```python
from build123d import *

# Parameters (mm, degrees)
SKETCH1_W           = 6.45
SKETCH1_H           = 14.9
SKETCH1_R           = 2.69
BOSS_EXTRUDE1_DEPTH = 2
SKETCH1_4_R         = 1.2
BOSS_EXTRUDE2_DEPTH = 1.08
SKETCH2_R           = 2.69
BOSS_EXTRUDE3_DEPTH = 3.45
BOSS_EXTRUDE4_DEPTH = 3.45
BOSS_EXTRUDE5_DEPTH = 2.45
SKETCH2_5_R         = 3.5
SKETCH2_5_R_2       = 2.69
BOSS_EXTRUDE6_DEPTH = 3.45
SKETCH2_6_R         = 3.5
SKETCH2_6_R_2       = 2.69
BOSS_EXTRUDE7_DEPTH = 5.5


with BuildPart() as part:
    # Sketch1 → Boss-Extrude1 (new body)
    with BuildSketch(Plane(origin=(0, 0, 0), x_dir=(1, 0, 0), z_dir=(0, 1, 0))):
        with BuildLine():
            ThreePointArc((-7.492590556, 11.885435909), (-7.808434164, 9.098816182), (-10.610710111, 9.209523926))
            Line((-10.610710111, 9.209523926), (-11.865304556, 10.471159095))
            ThreePointArc((-11.865304556, 10.471159095), (-15.824865609, 0.065218614), (-11.951209075, -10.373004706))
            Line((-11.951209075, -10.373004706), (-10.610710111, -9.209523926))
            ThreePointArc((-10.610710111, -9.209523926), (-7.808434164, -9.098816182), (-7.492590556, -11.885435909))
            Line((-7.492590556, -11.885435909), (-8.439163385, -13.386976745))
            ThreePointArc((-8.439163385, -13.386976745), (0, -15.825), (8.439163385, -13.386976745))
            Line((8.439163385, -13.386976745), (7.492590556, -11.885435909))
            ThreePointArc((7.492590556, -11.885435909), (7.808434164, -9.098816182), (10.610710111, -9.209523926))
            Line((10.610710111, -9.209523926), (11.865304556, -10.471159095))
            ThreePointArc((11.865304556, -10.471159095), (14.802011174, -5.597418173), (15.825, 0))
            ThreePointArc((15.825, 0), (14.802011174, 5.597418173), (11.865304556, 10.471159095))
            Line((11.865304556, 10.471159095), (10.610710111, 9.209523926))
            ThreePointArc((10.610710111, 9.209523926), (7.808434164, 9.098816182), (7.492590556, 11.885435909))
            Line((7.492590556, 11.885435909), (8.549217648, 13.316962965))
            ThreePointArc((8.549217648, 13.316962965), (0, 15.825), (-8.549217648, 13.316962965))
            Line((-8.549217648, 13.316962965), (-7.492590556, 11.885435909))
        make_face()
        with Locations((-8.77, 0)):
            Rectangle(SKETCH1_W, SKETCH1_H, mode=Mode.SUBTRACT)
        with Locations(Location((0, 0, 0), (0, 0, 270))):
            Circle(SKETCH1_R, mode=Mode.SUBTRACT)
        with Locations((8.77, 0)):
            Rectangle(SKETCH1_W, SKETCH1_H, mode=Mode.SUBTRACT)
    extrude(amount=BOSS_EXTRUDE1_DEPTH)

    # Sketch1_4 → Boss-Extrude2 (add)
    with BuildSketch(Plane(origin=(0, 0, 0), x_dir=(1, 0, 0), z_dir=(0, 1, 0))):
        with BuildLine():
            Line((-10.610710111, -9.209523926), (-11.951209075, -10.373004706))
            ThreePointArc((-11.951209075, -10.373004706), (-10.305960854, -12.009071399), (-8.439163385, -13.386976745))
            Line((-8.439163385, -13.386976745), (-7.492590556, -11.885435909))
            ThreePointArc((-7.492590556, -11.885435909), (-7.808434164, -9.098816182), (-10.610710111, -9.209523926))
        make_face()
        with Locations(Location((-9.15, -10.662082348, 0), (0, 0, 270))):
            Circle(SKETCH1_4_R, mode=Mode.SUBTRACT)
        with BuildLine():
            Line((-11.865304556, 10.471159095), (-10.610710111, 9.209523926))
            ThreePointArc((-10.610710111, 9.209523926), (-7.808434164, 9.098816182), (-7.492590556, 11.885435909))
            Line((-7.492590556, 11.885435909), (-8.549217648, 13.316962965))
            ThreePointArc((-8.549217648, 13.316962965), (-10.305960854, 12.009071399), (-11.865304556, 10.471159095))
        make_face()
        with Locations(Location((-9.15, 10.662082348, 0), (0, 0, 270))):
            Circle(SKETCH1_4_R, mode=Mode.SUBTRACT)
        with BuildLine():
            ThreePointArc((11.865304556, 10.471159095), (10.305960854, 12.009071399), (8.549217648, 13.316962965))
            Line((8.549217648, 13.316962965), (7.492590556, 11.885435909))
            ThreePointArc((7.492590556, 11.885435909), (7.808434164, 9.098816182), (10.610710111, 9.209523926))
            Line((10.610710111, 9.209523926), (11.865304556, 10.471159095))
        make_face()
        with Locations(Location((9.15, 10.662082348, 0), (0, 0, 270))):
            Circle(SKETCH1_4_R, mode=Mode.SUBTRACT)
        with BuildLine():
            Line((7.492590556, -11.885435909), (8.439163385, -13.386976745))
            ThreePointArc((8.439163385, -13.386976745), (10.256381074, -12.051442746), (11.865304556, -10.471159095))
            Line((11.865304556, -10.471159095), (10.610710111, -9.209523926))
            ThreePointArc((10.610710111, -9.209523926), (7.808434164, -9.098816182), (7.492590556, -11.885435909))
        make_face()
        with Locations(Location((9.15, -10.662082348, 0), (0, 0, 270))):
            Circle(SKETCH1_4_R, mode=Mode.SUBTRACT)
    extrude(amount=BOSS_EXTRUDE2_DEPTH)

    # Sketch2_3 → Boss-Extrude4 (add)
    with BuildSketch(Plane(origin=(0, 0, 0), x_dir=(1, 0, 0), z_dir=(0, 1, 0))):
        with BuildLine():
            Line((-8.549217648, 13.316962965), (-7.692058181, 12.155676285))
            ThreePointArc((-7.692058181, 12.155676285), (0, 14.385), (7.692058181, 12.155676285))
            Line((7.692058181, 12.155676285), (8.549217648, 13.316962965))
            ThreePointArc((8.549217648, 13.316962965), (0, 15.825), (-8.549217648, 13.316962965))
        make_face()
        with BuildLine():
            ThreePointArc((7.671239513, -12.168825307), (0, -14.385), (-7.671239513, -12.168825307))
            Line((-7.671239513, -12.168825307), (-8.439163385, -13.386976745))
            ThreePointArc((-8.439163385, -13.386976745), (0, -15.825), (8.439163385, -13.386976745))
            Line((8.439163385, -13.386976745), (7.671239513, -12.168825307))
        make_face()
    extrude(amount=-BOSS_EXTRUDE4_DEPTH)

    # Sketch2_4 → Boss-Extrude5 (add)
    with BuildSketch(Plane(origin=(0, 0, 0), x_dir=(1, 0, 0), z_dir=(0, 1, 0))):
        with BuildLine():
            Line((-11.995, -2.98), (-11.995, -1.63))
            Line((-11.995, -1.63), (-14.292351976, -1.63))
            ThreePointArc((-14.292351976, -1.63), (-14.198702945, -2.307609084), (-14.072946564, -2.98))
            Line((-14.072946564, -2.98), (-11.995, -2.98))
        make_face()
        with BuildLine():
            Line((-11.995, 1.63), (-11.995, 2.98))
            Line((-11.995, 2.98), (-14.072946564, 2.98))
            ThreePointArc((-14.072946564, 2.98), (-14.198702945, 2.307609084), (-14.292351976, 1.63))
            Line((-14.292351976, 1.63), (-11.995, 1.63))
        make_face()
        with BuildLine():
            Line((11.995, -2.98), (14.072946564, -2.98))
            ThreePointArc((14.072946564, -2.98), (14.198702945, -2.307609084), (14.292351976, -1.63))
            Line((14.292351976, -1.63), (11.995, -1.63))
            Line((11.995, -1.63), (11.995, -2.98))
        make_face()
        with BuildLine():
            ThreePointArc((14.292351976, 1.63), (14.198702945, 2.307609084), (14.072946564, 2.98))
            Line((14.072946564, 2.98), (11.995, 2.98))
            Line((11.995, 2.98), (11.995, 1.63))
            Line((11.995, 1.63), (14.292351976, 1.63))
        make_face()
    extrude(amount=-BOSS_EXTRUDE5_DEPTH)

    # Sketch2_5 → Boss-Extrude6 (add)
    with BuildSketch(Plane(origin=(0, 0, 0), x_dir=(1, 0, 0), z_dir=(0, 1, 0))):
        with Locations(Location((0, 0, 0), (0, 0, 270))):
            Circle(SKETCH2_5_R)
        with Locations(Location((0, 0, 0), (0, 0, 270))):
            Circle(SKETCH2_5_R_2, mode=Mode.SUBTRACT)
    extrude(amount=-BOSS_EXTRUDE6_DEPTH)



with BuildPart() as body_2:
    # Sketch2 → Boss-Extrude3 (new body)
    with BuildSketch(Plane(origin=(0, 0, 0), x_dir=(1, 0, 0), z_dir=(0, 1, 0))):
        with BuildLine():
            Line((-4.385, -3.5), (4.385, -3.5))
            Line((4.385, -3.5), (4.385, -8.61))
            Line((4.385, -8.61), (8.969561545, -8.61))
            ThreePointArc((8.969561545, -8.61), (9.85684589, -8.727148528), (10.610710111, -9.209523926))
            Line((10.610710111, -9.209523926), (11.865304556, -10.471159095))
            ThreePointArc((11.865304556, -10.471159095), (15.825, 0), (11.865304556, 10.471159095))
            Line((11.865304556, 10.471159095), (10.610710111, 9.209523926))
            ThreePointArc((10.610710111, 9.209523926), (9.85684589, 8.727148528), (8.969561545, 8.61))
            Line((8.969561545, 8.61), (4.385, 8.61))
            Line((4.385, 8.61), (4.385, 3.5))
            Line((4.385, 3.5), (-4.385, 3.5))
            Line((-4.385, 3.5), (-4.385, 8.61))
            Line((-4.385, 8.61), (-8.969561545, 8.61))
            ThreePointArc((-8.969561545, 8.61), (-9.85684589, 8.727148528), (-10.610710111, 9.209523926))
            Line((-10.610710111, 9.209523926), (-11.865304556, 10.471159095))
            ThreePointArc((-11.865304556, 10.471159095), (-15.824865609, 0.065218614), (-11.951209075, -10.373004706))
            Line((-11.951209075, -10.373004706), (-10.610710111, -9.209523926))
            ThreePointArc((-10.610710111, -9.209523926), (-9.85684589, -8.727148528), (-8.969561545, -8.61))
            Line((-8.969561545, -8.61), (-4.385, -8.61))
            Line((-4.385, -8.61), (-4.385, -3.5))
        make_face()
        with BuildLine():
            Line((-5.545, 7.45), (-5.545, 1.63))
            Line((-5.545, 1.63), (-3.795, 1.63))
            Line((-3.795, 1.63), (-3.795, -1.63))
            Line((-3.795, -1.63), (-5.545, -1.63))
            Line((-5.545, -1.63), (-5.545, -7.45))
            Line((-5.545, -7.45), (-12.30551604, -7.45))
            ThreePointArc((-12.30551604, -7.45), (-14.385, 0), (-12.30551604, 7.45))
            Line((-12.30551604, 7.45), (-5.545, 7.45))
        make_face(mode=Mode.SUBTRACT)
        with BuildLine():
            Line((3.795, -1.63), (3.795, 1.63))
            Line((3.795, 1.63), (5.545, 1.63))
            Line((5.545, 1.63), (5.545, 7.45))
            Line((5.545, 7.45), (12.30551604, 7.45))
            ThreePointArc((12.30551604, 7.45), (14.385, 0), (12.30551604, -7.45))
            Line((12.30551604, -7.45), (5.545, -7.45))
            Line((5.545, -7.45), (5.545, -1.63))
            Line((5.545, -1.63), (3.795, -1.63))
        make_face(mode=Mode.SUBTRACT)
        with Locations(Location((0, 0, 0), (0, 0, 270))):
            Circle(SKETCH2_R, mode=Mode.SUBTRACT)
    extrude(amount=-BOSS_EXTRUDE3_DEPTH)


with BuildPart() as part_1:
    add(part.part)

    add(body_2.part)  # Boss-Extrude7 merges body 2
    # Sketch2_6 → Boss-Extrude7 (add)
    with BuildSketch(Plane(origin=(0, 0, 0), x_dir=(1, 0, 0), z_dir=(0, 1, 0))):
        Circle(SKETCH2_6_R)
        with Locations(Location((0, 0, 0), (0, 0, 270))):
            Circle(SKETCH2_6_R_2, mode=Mode.SUBTRACT)
        with BuildLine():
            Line((3.795, 3.5), (0, 3.5))
            ThreePointArc((0, 3.5), (2.474873734, 2.474873734), (3.5, 0))
            ThreePointArc((3.5, 0), (2.474873734, -2.474873734), (0, -3.5))
            Line((0, -3.5), (3.795, -3.5))
            Line((3.795, -3.5), (3.795, -1.63))
            Line((3.795, -1.63), (3.795, 1.63))
            Line((3.795, 1.63), (3.795, 3.5))
        make_face()
        with BuildLine():
            Line((-3.795, 3.5), (-3.795, 1.63))
            Line((-3.795, 1.63), (-3.795, -1.63))
            Line((-3.795, -1.63), (-3.795, -3.5))
            Line((-3.795, -3.5), (0, -3.5))
            ThreePointArc((0, -3.5), (-3.5, 0), (0, 3.5))
            Line((0, 3.5), (-3.795, 3.5))
        make_face()
    extrude(amount=-BOSS_EXTRUDE7_DEPTH)


solid = part_1.part
```
The listing builds one solid part. Answer for the finished solid, in the listing's coordinates (mm). A direction names the side the tool comes from. Coordinates: 2 decimals unless noted, no trailing zeros. Loops run counter-clockwise (first coordinate to the right, second up) from the corner with the lowest first, then second, coordinate; pieces in that order, holes last. Notation, with made-up numbers: M 12.5,20 L 68.5,20 A32 cw 68.5,53 Z; hole C 50,35 d3. An arc over 180 degrees is marked long. Answer as CSV lines item,"result". Start each with the question number.
(1) The part is cut by section D-D (z = -0.5). Give the vertices of the cut face in (x, y) (3 decimals), and give its area (3 significant figures).
(2) The mould has two halves that part along Z. Classify faces 5 (the flat face through (9, -1, 7.45)), 6 (the flat face through (-11.29, 1.53, 9.8)), 7 (the cylindrical face through (9.87, -1.7, -8.73)), 8 (the flat face through (-4.385, -2, 6)): pulls with the +Z half, pulls with the -Z half, needs draft (parallel to the pull), parting line crosses it, or undercut.
(3) The part is cut by section C-C (y = -1.75). State how many separate pieces and enclosed holes the cut face has, and give its area (3 significant figures).
(4) The part is cut by section B-B (z = -10). Give the vertices of the cut face in (x, y), and give its area (3 significant figures).
(5) The part is cut by section A-A (y = -4). Give the vertices of the cut face in (x, z) (3 decimals).
(6) Given pin 1 (3 mm diameter, centred on y = -2.5, z = -4, fed in from -X); pin 2 (3 mm diameter, centred on x = -6.5, z = -6, fed in from -Y); pin 3 (3 mm diameter, centred on x = -11, y = 0, fed in from +Z); pin 4 (3.5 mm diameter, centred on x = 10, z = 4.5, fed in from -Y), each flat-ended and moving along its own axis, determine where each tip first touches the part or whether it passes through.
(7) Find the intervals of material crossed by L1, parallel to X at y = 1.3, z = 0 (3 decimals); L2, parallel to Z at x = 9, y = -1; L3, parallel to X at y = -1.75, z = -4 (3 decimals), in increasing order. Write a range as [from, to].
(8) For faces 1 (the flat face through (-7.96, 1.53, 12.63)), 2 (the flat face through (11.995, 1, 0)), 3 (the flat face through (8.115, -1.701, -12.728)), 4 (the flat face through (-13, 0, 0)), determine the directions among +Z, -Z, +X, -X, +Y, -Y from which every point of the face is accessible in a straight line to the end or side of a thin tool.
Determined:
1,outline,"M -15.817,-3.45 L -14.376,-3.45 L -14.376,0 L -11.995,0 L -11.995,2 L -15.817,2 Z; M -5.545,0 L -3.795,0 L -3.795,-5.5 L -2.643,-5.5 L -2.643,2 L -5.545,2 Z; M 2.643,-5.5 L 3.795,-5.5 L 3.795,0 L 5.545,0 L 5.545,2 L 2.643,2 Z; M 11.995,0 L 14.376,0 L 14.376,-3.45 L 15.817,-3.45 L 15.817,2 L 11.995,2 Z"
1,area,"49.5 mm2"
2,face 5,"undercut"
2,face 6,"pulls with the +Z half"
2,face 7,"pulls with the -Z half"
2,face 8,"undercut"
3,separate pieces,"3"
3,enclosed holes,"3"
3,area,"223 mm2"
4,outline,"M -12.27,-3.45 L -11.4,-3.45 L -11.4,0 L -10.15,0 L -10.15,1.08 L -11.4,1.08 L -11.4,2 L -12.27,2 Z; M -8.15,0 L 8.15,0 L 8.15,1.08 L 7.2,1.08 L 7.2,2 L -7.2,2 L -7.2,1.08 L -8.15,1.08 Z; M 10.15,0 L 11.4,0 L 11.4,-3.45 L 12.27,-3.45 L 12.27,2 L 11.4,2 L 11.4,1.08 L 10.15,1.08 Z"
4,area,"43.0 mm2"
5,outline,"M -3.795,-3.5 L 3.795,-3.5 L 3.795,3.5 L -3.795,3.5 Z; hole C 0,0 d5.38"
6,pin 1,"x = -15.63"
6,pin 2,"y = -3.45"
6,pin 3,"z = 12.66"
6,pin 4,"through"
7,L1,"[-15.825, -11.995], [-5.545, -2.69], [2.69, 5.545], [11.995, 15.825]"
7,L2,"[-8.61, -7.45], [7.45, 8.61]"
7,L3,"[-15.311, -13.818], [-5.545, -4.385], [4.385, 5.545], [13.818, 15.311]"
8,face 1,"-X, +Y"
8,face 2,"+Y, -Y"
8,face 3,"+X, -Y"
8,face 4,"-Y"
